Check sheet for the modelled part. Datum: model origin and axes. Units: mm. Face numbers are marked on the shaded views. A direction names the side the tool comes from. Coordinates: 2 decimals unless noted, no trailing zeros. Loops run counter-clockwise (first coordinate to the right, second up) from the corner with the lowest first, then second, coordinate; pieces in that order, holes last. Notation, with made-up numbers: M 23.5,55.25 L 60.5,55.25 A15 cw 60.5,70.25 Z; hole C 43.25,88.5 d10. An arc over 180 degrees is marked long. Write each question's results on one line, items separated by ' | '. Start each with the question number.
from build123d import *

# Parameters (mm, degrees)
SKETCH3_R               = 53.4
BOSS_EXTRUDE1_DEPTH     = 38.5
SKETCH4_R               = 8
CUT_EXTRUDE1_DEPTH      = 85.766561804
BOSS_EXTRUDE3_START     = 2
SKETCH6_R               = 16
SKETCH6_R_2             = 8
BOSS_EXTRUDE3_DEPTH     = 2
SKETCH8_R               = 2.5
CUT_EXTRUDE4_DEPTH      = 20
SKETCH9_R               = 53.4
SKETCH9_R_2             = 45
CUT_EXTRUDE5_DEPTH      = 34.5
CUT_EXTRUDE6_DEPTH      = 2
CUT_EXTRUDE6_DEPTH_BACK = 5
SKETCH10_R              = 50
SKETCH11_R              = 30
CUT_EXTRUDE7_DEPTH      = 10


with BuildPart() as part:
    # Sketch3 → Boss-Extrude1 (new body)
    with BuildSketch(Plane.XY):
        Circle(SKETCH3_R)
    extrude(amount=-BOSS_EXTRUDE1_DEPTH)

    # Sketch4 → Cut-Extrude1 (cut, through all)
    with BuildSketch(Plane.XY):
        Circle(SKETCH4_R)
    extrude(amount=-CUT_EXTRUDE1_DEPTH, mode=Mode.SUBTRACT)

    # Sketch6 → Boss-Extrude3 (add)
    with BuildSketch(Plane.XY.offset(BOSS_EXTRUDE3_START)):
        Circle(SKETCH6_R)
        Circle(SKETCH6_R_2, mode=Mode.SUBTRACT)
    extrude(amount=-BOSS_EXTRUDE3_DEPTH)

    # Sketch8 → Cut-Extrude4 (cut)
    with BuildSketch(Plane(origin=(0, 0, -38.5), x_dir=(-1, 0, 0), z_dir=(0, 0, -1))):
        with Locations((0, 30)):
            Circle(SKETCH8_R)
        with Locations((30, 0)):
            Circle(SKETCH8_R)
        with Locations((0, -30)):
            Circle(SKETCH8_R)
        with Locations((-30, 0)):
            Circle(SKETCH8_R)
    extrude(amount=-CUT_EXTRUDE4_DEPTH, mode=Mode.SUBTRACT)

    # Sketch9 → Cut-Extrude5 (cut)
    with BuildSketch(Plane.XY):
        Circle(SKETCH9_R)
        Circle(SKETCH9_R_2, mode=Mode.SUBTRACT)
    extrude(amount=-CUT_EXTRUDE5_DEPTH, mode=Mode.SUBTRACT)

    # Sketch10 → Cut-Extrude6 (cut, two sides: drawn at the far end of the back side and taken through both)
    with BuildSketch(Plane.XY.offset(-CUT_EXTRUDE6_DEPTH_BACK)):
        Circle(SKETCH10_R)
    extrude(amount=CUT_EXTRUDE6_DEPTH + CUT_EXTRUDE6_DEPTH_BACK, mode=Mode.SUBTRACT)

    # Sketch11 → Cut-Extrude7 (cut)
    with BuildSketch(Plane.XY.offset(-5)):
        Circle(SKETCH11_R)
    extrude(amount=-CUT_EXTRUDE7_DEPTH, mode=Mode.SUBTRACT)


solid = part.part
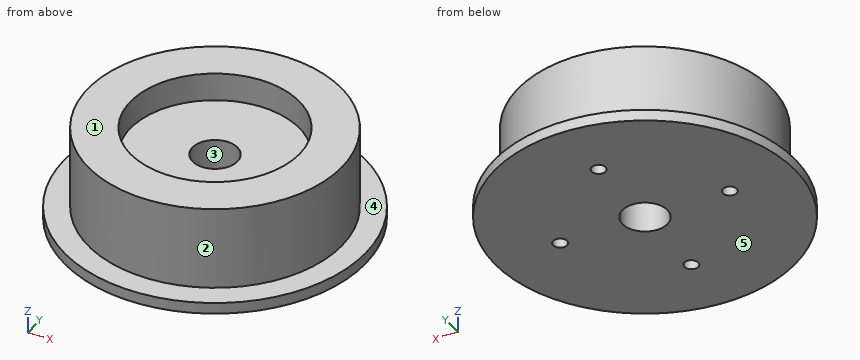
Item 1: Release check for a two-part mould opening along Y. For the marked faces 1, 2 and 3 record: +Y half, -Y half, draft (parallel to the pull), parting line (faces both ways), or undercut.
Item 2: Section check D-D (z = -17). Record the cut outline in (x, y), plus the area to 3 significant figures.
Item 3: Depth check by flat-ended pin: P1, Ø8, axis at x = -11.5, y = -27.5, coming from the +Z side; P2, Ø14.5, axis at x = 0, y = 0, coming from the +Z side (3 decimals); P3, Ø8, axis at y = 33, z = -20, coming from the -X side; P4, Ø3, axis at x = 4, z = -22, coming from the +Y side. Enter the tip coordinate at first touch or a pass-through.
Item 4: Section check A-A (x = 0). Record the cut outline in (y, z).
Item 5: Section check C-C (z = -28). Record the cut outline in (x, y), plus the area to 3 significant figures.
Item 6: Tool access check on the marked faces 4 and 5. Record the directions out of +Z, -Z, +X, -X, +Y, -Y that give a thin tool (end or side, any length) a straight path to the whole face; none if there is none.
Item 7: Thickness scan on line 1 (Y direction, x = 0, z = -24); line 2 (Y direction, x = 2, z = -26); line 3 (Y direction, x = 0, z = -13). Record the ranges inside material, lowest first.
Computed values:
1) face 1: draft | face 2: parting line | face 3: undercut
2) outline: C 0,0 d90; hole C 0,0 d16 | area: 6,160 mm²
3) P1: stops at z = -5 | P2: passes through | P3: stops at x = -34.41 | P4: stops at y = 44.93
4) outline: M -53.4,-38.5 L -32.5,-38.5 L -32.5,-18.5 L -27.5,-18.5 L -27.5,-38.5 L -8,-38.5 L -8,-15 L -30,-15 L -30,-5 L -45,-5 L -45,-34.5 L -53.4,-34.5 Z; M 8,-38.5 L 27.5,-38.5 L 27.5,-18.5 L 32.5,-18.5 L 32.5,-38.5 L 53.4,-38.5 L 53.4,-34.5 L 45,-34.5 L 45,-5 L 30,-5 L 30,-15 L 8,-15 Z
5) outline: C 0,0 d90; hole C -30,0 d5; hole C 0,0 d16; hole C 0,-30 d5; hole C 0,30 d5; hole C 30,0 d5 | area: 6,080 mm²
6) face 4: +Z | face 5: -Z, +X, -X, +Y, -Y
7) line 1: y = -45 to -32.5, -27.5 to -8, 8 to 27.5, 32.5 to 45 | line 2: y = -44.96 to -31.5, -28.5 to -7.75, 7.75 to 28.5, 31.5 to 44.96 | line 3: y = -45 to -30, 30 to 45
